```python
from build123d import *

# Parameters (mm, degrees)
BOSS_EXTRUDE1_DEPTH                          = 61.6
BOSS_EXTRUDE3_DEPTH                          = 97.007351
SKETCH3_R                                    = 42.5
CUT_EXTRUDE1_DEPTH                           = 53.5
BOSS_EXTRUDE2_START                          = 8.1
BOSS_EXTRUDE2_DEPTH                          = 31.22
CBORE_FOR_M5_HEX_HEAD_CAP_SCREW1_D           = 4.4
CBORE_FOR_M5_HEX_HEAD_CAP_SCREW1_DEPTH       = 5.5
CBORE_FOR_M5_HEX_HEAD_CAP_SCREW1_CBORE_D     = 4.6
CBORE_FOR_M5_HEX_HEAD_CAP_SCREW1_CBORE_DEPTH = 0.6
CBORE_FOR_M5_HEX_HEAD_CAP_SCREW1_TIP         = 1.321893362
CUT_EXTRUDE3_DEPTH                           = 45
BOSS_EXTRUDE4_REACH                          = 168.648
CUT_EXTRUDE2_REACH                           = 130.328
SKETCH6_W                                    = 20.5
SKETCH6_H                                    = 21
CUT_EXTRUDE2_DIRECTION_2_DEPTH               = 40
SKETCH13_W                                   = 20
SKETCH13_H                                   = 10
CUT_EXTRUDE4_DEPTH                           = 6


with BuildPart() as part:
    # Sketch1 → Boss-Extrude1 (new body)
    with BuildSketch(Plane(origin=(0, 0, 0), x_dir=(1, 0, 0), z_dir=(0, 1, 0))):
        Polygon((-48.503675457, 20.090880199), (-48.503675457, -20.090880199), (-20.090880199, -48.503675457), (20.090880199, -48.503675457), (48.503675457, -20.090880199), (48.503675457, 20.090880199), (20.090880199, 48.503675457), (-20.090880199, 48.503675457), align=None)
    extrude(amount=BOSS_EXTRUDE1_DEPTH)

    # Sketch10 → Boss-Extrude3 (add, through all)
    with BuildSketch(Plane.XY.offset(48.503675457)):
        Polygon((-20.090880199, 0), (-110.090880199, 0), (-120.692155197, 39.564496916), (-120.692155197, 49.564496916), (-65.692155197, 49.564496916), (-48.503675457, 61.6), (-20.090880199, 61.6), align=None)
    extrude(amount=-BOSS_EXTRUDE3_DEPTH)

    # Sketch3 → Cut-Extrude1 (cut)
    with BuildSketch(Plane(origin=(0, 61.6, 0), x_dir=(1, 0, 0), z_dir=(0, 1, 0))):
        with Locations(Location((0, 0, 0), (0, 0, 270))):
            Circle(SKETCH3_R)
    extrude(amount=-CUT_EXTRUDE1_DEPTH, mode=Mode.SUBTRACT)

    # Sketch5 → Boss-Extrude2 (add)
    with BuildSketch(Plane(origin=(0, 0, 0), x_dir=(1, 0, 0), z_dir=(0, 1, 0)).offset(BOSS_EXTRUDE2_START)):
        Polygon((41.245454295, -10.25), (38.9, -10.25), (38.9, 29.694555656), (29.9, 29.694555656), (29.9, -10.25), (-10.1, -10.25), (-10.1, 41.282441788), (-19.1, 41.282441788), (-19.1, -10.25), (-41.245454295, -10.25), (-41.245454295, -19.25), (-19.1, -19.25), (-19.1, -41.282441788), (-10.1, -41.282441788), (-10.1, -19.25), (29.9, -19.25), (29.9, -29.694555656), (38.9, -29.694555656), (38.9, -19.25), (41.245454295, -19.25), align=None)
    extrude(amount=BOSS_EXTRUDE2_DEPTH)

    # CBORE for M5 Hex Head Cap Screw1
    with Locations(Plane(origin=(0, 39.32, 0), x_dir=(1, 0, 0), z_dir=(0, 1, 0))):
        with Locations((-14.85, -5), (-14.85, 5), (34.65, 5), (34.65, -5)):
            CounterBoreHole(CBORE_FOR_M5_HEX_HEAD_CAP_SCREW1_D / 2, CBORE_FOR_M5_HEX_HEAD_CAP_SCREW1_CBORE_D / 2, CBORE_FOR_M5_HEX_HEAD_CAP_SCREW1_CBORE_DEPTH, depth=CBORE_FOR_M5_HEX_HEAD_CAP_SCREW1_DEPTH)
            with Locations((0, 0, -(CBORE_FOR_M5_HEX_HEAD_CAP_SCREW1_DEPTH + CBORE_FOR_M5_HEX_HEAD_CAP_SCREW1_TIP / 2))):  # 118° drill point
                Cone(0, CBORE_FOR_M5_HEX_HEAD_CAP_SCREW1_D / 2, CBORE_FOR_M5_HEX_HEAD_CAP_SCREW1_TIP, mode=Mode.SUBTRACT)

    # Sketch11 → Cut-Extrude3 (cut)
    with BuildSketch(Plane(origin=(0, 61.6, 0), x_dir=(1, 0, 0), z_dir=(0, 1, 0))):
        Polygon((-52.5, 21.746212025), (-52.5, -21.746212025), (-31.742536568, -42.503675457), (-114.692155197, -42.503675457), (-114.692155197, 42.503675457), (-31.742536568, 42.503675457), align=None)
    extrude(amount=-CUT_EXTRUDE3_DEPTH, mode=Mode.SUBTRACT)

    # Sketch12 → Boss-Extrude4 (add, up to next)
    with BuildSketch(Plane.XY.offset(48.503675457), mode=Mode.PRIVATE) as boss_extrude4_sk1:
        Polygon((-110.090880199, 0), (-104.090880199, 0), (-114.692155197, 39.564496916), (-120.692155197, 39.564496916), align=None)
    boss_extrude4_tool1 = extrude(boss_extrude4_sk1.sketch, amount=-BOSS_EXTRUDE4_REACH, mode=Mode.PRIVATE) - part.part
    add(boss_extrude4_tool1.solids().sort_by_distance((-112.391518, 19.782248, 48.503675))[0])

    # Sketch6 → Cut-Extrude2 (cut, up to next)
    with BuildSketch(Plane.ZY.offset(19.1), mode=Mode.PRIVATE) as cut_extrude2_sk1:
        with Locations((0, 18.6)):
            Rectangle(SKETCH6_W, SKETCH6_H)
    cut_extrude2_tool1 = extrude(cut_extrude2_sk1.sketch, amount=-CUT_EXTRUDE2_REACH, mode=Mode.PRIVATE) & part.part
    add(cut_extrude2_tool1.solids().sort_by_distance((-19.1, 18.6, 0))[0], mode=Mode.SUBTRACT)

    # Sketch6 → Cut-Extrude2 direction 2 (cut)
    with BuildSketch(Plane.ZY.offset(19.1)):
        with Locations((0, 18.6)):
            Rectangle(SKETCH6_W, SKETCH6_H)
    extrude(amount=CUT_EXTRUDE2_DIRECTION_2_DEPTH, mode=Mode.SUBTRACT)

    # Sketch13 → Cut-Extrude4 (cut)
    with BuildSketch(Plane(origin=(0, 0, -48.503675457), x_dir=(-1, 0, 0), z_dir=(0, 0, -1))):
        with Locations((95.692155197, 20)):
            Rectangle(SKETCH13_W, SKETCH13_H)
    extrude(amount=-CUT_EXTRUDE4_DEPTH, mode=Mode.SUBTRACT)


solid = part.part
```
Build history of the part. All positions in model axes, mm. A direction names the side the tool comes from. Coordinates: 2 decimals unless noted, no trailing zeros. Write each loop counter-clockwise with the first axis right and the second up, starting at its lowest first coordinate (ties: lowest second). Pieces come first, ordered by that corner, then holes.
1. Pull direction Z, two halves, no side cores. Call faces 6 (the flat face through (-14, 23, 10.25)), 7 (the flat face through (-105.692, 20, -46)), 8 (the flat face through (-49, 31, 48.504)): released by +Z, released by -Z, zero draft, split by the parting line, or undercut.
Answer block:
face 6: undercut
face 7: zero draft
face 8: released by +Z
2. Band-saw the part on C-C, the plane y = 55. Give the cut face in (x, z), and give its area (3 significant figures).
Answer block:
outline: (-57.93, -48.5) - (20.09, -48.5) - (48.5, -20.09) - (48.5, 20.09) - (20.09, 48.5) - (-57.93, 48.5) - (-57.93, 42.5) - (-31.74, 42.5) - (-52.5, 21.75) - (-52.5, -21.75) - (-31.74, -42.5) - (-57.93, -42.5) - close; hole circle Ø85 at (0, 0)
area: 2,950 mm2
3. 3-axis set-ups, long thin cutter, end or side, ignore diameter. For faces 1 (the flat face through (40, 8.1, -1)), 2 (the flat face through (-96, 25, -46)), 3 (the flat face through (-116, 49.564, 0)), 4 (the flat face through (34.098, 30.369, 34.496)), 5 (the flat face through (-120.692, 44, 1)): which of +Z, -Z, +X, -X, +Y, -Y reach the whole face in a straight line?
Answer block:
face 1: +Y
face 2: -Z
face 3: +Z, -Z, -X, +Y
face 4: +Z, +X, +Y, -Y
face 5: +Z, -Z, -X, +Y, -Y
4. Band-saw the part on B-B, the plane y = 27. Give the number of separate pieces and of enclosed holes in the cut face, and give its area (3 significant figures).
Answer block:
separate pieces: 1
enclosed holes: 4
area: 5,490 mm2
5. Drill centre lines: probe 1 along Z at (x, y) = (-14.85, 39.2); probe 2 along Z at (x, y) = (-54.5, 47); probe 3 along Z at (x, y) = (-14, 34). Where is each one in solid material? Low to high.
Answer block:
probe 1: z = -48.5 to -7.3, -2.7 to 2.7, 7.3 to 48.5
probe 2: z = -48.5 to -42.5, 42.5 to 48.5
probe 3: z = -48.5 to -7.03, -2.97 to 2.97, 7.03 to 48.5
6. Drop flat-ended pins along their axis: pin 1 (9 mm diameter, centred on x = -46.5, z = -3, fed in from -Y); pin 2 (20.5 mm diameter, centred on y = 16, z = 26, fed in from -X); pin 3 (10 mm diameter, centred on x = -10.5, z = -16.5, fed in from +Y); pin 4 (5 mm diameter, centred on x = -61.5, z = -36.5, fed in from +Y). Give the stop position or say it passes through.
Answer block:
pin 1: stops at y = 0
pin 2: stops at x = -117.12
pin 3: stops at y = 39.32
pin 4: stops at y = 16.6
7. Band-saw the part on A-A, the plane x = -68.5. Give the cut face in (y, z).
Answer block:
outline: (0, -48.5) - (49.56, -48.5) - (49.56, -42.5) - (16.6, -42.5) - (16.6, 42.5) - (49.56, 42.5) - (49.56, 48.5) - (0, 48.5) - close
